Here's the drawing with two shaded views (mm, measured from the low corner). I have some questions. A direction names the side the tool comes from. Round coordinates to 2 decimals unless told otherwise and drop trailing zeros. Loops run counter-clockwise (first coordinate to the right, second up) from the corner with the lowest first, then second, coordinate; pieces in that order, holes last. Notation, with made-up numbers: M 10.5,62 L 18.5,62 A20 ccw 18.5,88 Z; hole C 24.5,-14.75 d9. An arc over 180 degrees is marked long. Write each question's results on one line, items separated by ' | '. Start each with the question number.
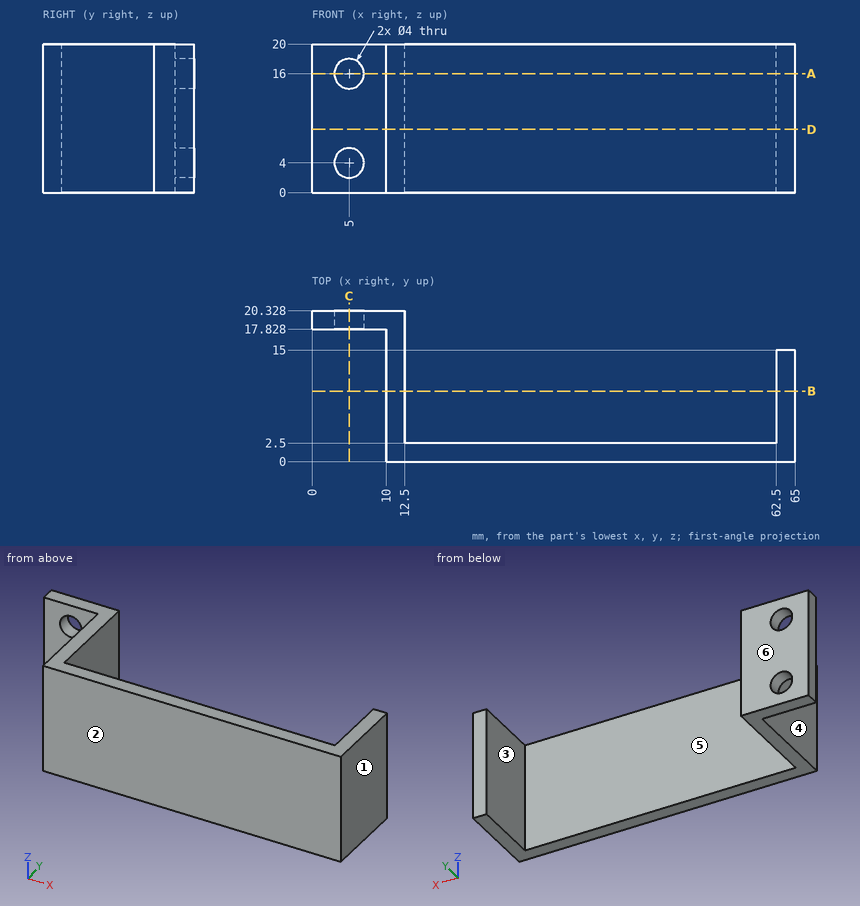
Item 1: If we section it at D-D on z = 8.5: Please give me the cut outline in (x, y), and give its area (3 significant figures).
Item 2: If we section it at A-A on z = 16: Please give me the cut outline in (x, y), and give its area (3 significant figures).
Item 3: I'm going to push flat-ended pins straight in: pin 1 (4.5 mm diameter, centred on x = 5, z = 16, fed in from -Y); pin 2 (5 mm diameter, centred on y = 12.5, z = 14.5, fed in from -X); pin 3 (10 mm diameter, centred on y = 17, z = 7.5, fed in from -X); pin 4 (0.8 mm diameter, centred on x = 63, z = 9.5, fed in from +Y). Where does each tip first touch, or does it pass through?
Item 4: If we section it at B-B on y = 9.5: Please give me the cut outline in (x, z), and give its area (3 significant figures).
Item 5: I need wall thicknesses on L1, parallel to Z at x = 5, y = 19.1; L2, parallel to X at y = 4, z = 8.5; L3, parallel to X at y = 2.25, z = 4.75. Which ranges of each line are inside material? Lowest first, please.
Item 6: If we section it at C-C on x = 5: Please give me the cut outline in (y, z).
Item 7: If we mould it in two halves opening along X, with no side actions, what happens to the marked faces 1, 2 and 3? For each: released by +X, released by -X, zero draft, split by the parting line, or undercut.
Item 8: Which directions (+Z, -Z, +X, -X, +Y, -Y) give clear straight access to the entire face, cutting with the end or side of a thin tool? Please do the marked faces 4, 5 and 6.
Numbers:
1) outline: M 0,17.83 L 10,17.83 L 10,0 L 65,0 L 65,15 L 62.5,15 L 62.5,2.5 L 12.5,2.5 L 12.5,20.33 L 0,20.33 Z | area: 238 mm²
2) outline: M 0,17.83 L 3,17.83 L 3,20.33 L 0,20.33 Z; M 7,17.83 L 10,17.83 L 10,0 L 65,0 L 65,15 L 62.5,15 L 62.5,2.5 L 12.5,2.5 L 12.5,20.33 L 7,20.33 Z | area: 228 mm²
3) pin 1: y = 17.83 | pin 2: x = 10 | pin 3: x = 0 | pin 4: y = 15
4) outline: M 10,0 L 12.5,0 L 12.5,20 L 10,20 Z; M 62.5,0 L 65,0 L 65,20 L 62.5,20 Z | area: 100 mm²
5) L1: 0 to 2, 6 to 14, 18 to 20 | L2: 10 to 12.5, 62.5 to 65 | L3: 10 to 65
6) outline: M 17.83,0 L 20.33,0 L 20.33,2 L 17.83,2 Z; M 17.83,6 L 20.33,6 L 20.33,14 L 17.83,14 Z; M 17.83,18 L 20.33,18 L 20.33,20 L 17.83,20 Z
7) face 1: released by +X | face 2: zero draft | face 3: undercut
8) face 4: +Z, -Z, -X, -Y | face 5: +Z, -Z, +Y | face 6: +Z, -Z, +X, -X, +Y
